The model under review builds one solid part; all positions refer to its coordinate system, in mm. A direction names the side the tool comes from. Coordinates: 2 decimals unless noted, no trailing zeros. Loops run counter-clockwise (first coordinate to the right, second up) from the corner with the lowest first, then second, coordinate; pieces in that order, holes last. Notation, with made-up numbers: M -29,-29.5 L -1,-29.5 A23 cw -1,-18.5 Z; hole C 56.5,15 d9. An arc over 180 degrees is marked long. Return JSON: item names as keys, results as strings.
```python
from build123d import *

# Parameters (mm, degrees)
SKETCH1_W           = 139.7
SKETCH1_H           = 171.45
BOSS_EXTRUDE1_DEPTH = 2.54
CUT_EXTRUDE1_DEPTH  = 2.54
SKETCH12_R          = 1.46685
CUT_EXTRUDE6_DEPTH  = 3.54
SKETCH24_R          = 5.075
BOSS_EXTRUDE8_DEPTH = 33
FILLET2_R           = 2
SKETCH26_R          = 2.25
CUT_EXTRUDE16_DEPTH = 5


with BuildPart() as part:
    # Sketch1 → Boss-Extrude1 (new body)
    with BuildSketch(Plane.XY):
        with Locations((-69.85, 85.725)):
            Rectangle(SKETCH1_W, SKETCH1_H)
    extrude(amount=BOSS_EXTRUDE1_DEPTH)

    # Sketch3 → Cut-Extrude1 (cut)
    with BuildSketch(Plane.XY.offset(2.54)):
        Polygon((-28.321, 12.065), (-9.906, 12.065), (-9.906, 3.683), (-68.326, 3.683), (-68.326, 12.065), (-54.991, 12.065), (-54.991, 28.575), (-49.911, 28.575), (-28.321, 28.575), align=None)
    extrude(amount=-CUT_EXTRUDE1_DEPTH, mode=Mode.SUBTRACT)

    # Sketch12 → Cut-Extrude6 (cut, through all)
    with BuildSketch(Plane.XY.offset(2.54)):
        with Locations((-134.62, 5.08)):
            Circle(SKETCH12_R)
        with Locations((-134.62, 166.37)):
            Circle(SKETCH12_R)
        with Locations((-5.08, 166.37)):
            Circle(SKETCH12_R)
        with Locations((-5.08, 5.08)):
            Circle(SKETCH12_R)
    extrude(amount=-CUT_EXTRUDE6_DEPTH, mode=Mode.SUBTRACT)

    # Sketch24 → Boss-Extrude8 (add)
    with BuildSketch(Plane.XY.offset(2.54)):
        with Locations((-72.633345717, 111.8489)):
            Circle(SKETCH24_R)
    extrude(amount=BOSS_EXTRUDE8_DEPTH)

    # Fillet2
    fillet2_edges = [part.edges().sort_by_distance(p)[0] for p in [
        (-77.708345717, 111.8489, 2.54),
    ]]
    fillet(fillet2_edges, radius=FILLET2_R)

    # Sketch26 → Cut-Extrude16 (cut)
    with BuildSketch(Plane.XY.offset(35.54)):
        with Locations((-72.633345717, 111.8489)):
            Circle(SKETCH26_R)
    extrude(amount=-CUT_EXTRUDE16_DEPTH, mode=Mode.SUBTRACT)


solid = part.part
```
1. The part is to be moulded in two halves that separate along Y. For faces 3 (the face through (-71, 87, 2.54)), 4 (the face through (-70.292, 107.347, 19.823)), 5 (the face through (-74.88, 111.95, 33.08)), say which applies: released by +Y, released by -Y, zero draft, split by the parting line, or undercut.
Check values:
{"face 3": "zero draft", "face 4": "split by the parting line", "face 5": "undercut"}
2. Machinability: for faces 1 (the face through (-70, 111, 35.54)), 2 (the face through (-73, 112, 30.54)), which of the approach directions +Z, -Z, +X, -X, +Y, -Y give a long, thin tool a straight path to every point of the face, cutting with its end or side? Answer none if there is none.
Check values:
{"face 1": "+Z, +X, -X, +Y, -Y", "face 2": "+Z"}
3. Add section D-D on z = 32.5. Give the boundary of the cut face in (x, y) (3 decimals), plus the area to 3 significant figures.
Check values:
{"outline": "C -72.633,111.849 d10.15; hole C -72.633,111.849 d4.5", "area": "65.0 mm²"}
4. Add section C-C on x = -127. Give the boundary of the cut face in (y, z).
Check values:
{"outline": "M 0,0 L 171.45,0 L 171.45,2.54 L 0,2.54 Z"}
5. Add section B-B on y = 45.5. Give the boundary of the cut face in (x, z), plus the area to 3 significant figures.
Check values:
{"outline": "M -139.7,0 L 0,0 L 0,2.54 L -139.7,2.54 Z", "area": "355 mm²"}
6. Add section A-A on x = -33. Give the boundary of the cut face in (y, z) (3 decimals), plus the area to 3 significant figures.
Check values:
{"outline": "M 0,0 L 3.683,0 L 3.683,2.54 L 0,2.54 Z; M 28.575,0 L 171.45,0 L 171.45,2.54 L 28.575,2.54 Z", "area": "372 mm²"}
7. To check wall thickness, follow line 1 (Y direction, x = -134.62, z = 1.4); line 2 (X direction, y = 166.37, z = 1.95); line 3 (Z direction, x = -22, y = 121). State the ranges of each line that lie inside material, in increasing order.
Check values:
{"line 1": "0 to 3.61, 6.55 to 164.9, 167.84 to 171.45", "line 2": "-139.7 to -136.09, -133.15 to -6.55, -3.61 to 0", "line 3": "0 to 2.54"}
8. Insertion check: pin 1 Ø3.5 at (x, y) = (-5.08, 5.08) entering from +Z; pin 2 Ø2.5 at (x, y) = (-134.62, 166.37) entering from +Z; pin 3 Ø2.5 at (x, y) = (-72.63, 111.85) entering from +Z; pin 4 Ø5 at (x, z) = (-72, 30.5) entering from +Y. Each pin has a flat end and moves straight along its axis. Give the tip position at first contact, or say it passes through.
Check values:
{"pin 1": "z = 2.54", "pin 2": "through", "pin 3": "z = 30.54", "pin 4": "y = 116.92"}
